Read the model definition and answer for the solid it produces. Units are mm, in the model's axes. A direction names the side the tool comes from. Give positions to 0.01 mm unless a question says otherwise; leave off trailing zeros. Write each loop counter-clockwise with the first axis right and the second up, starting at its lowest first coordinate (ties: lowest second). Pieces come first, ordered by that corner, then holes. Notation, with made-up numbers: (35, 9) - (65, 9) arc R13 ccw to (65, 16) - close; hole circle Ø3 at (-34, 65.5). An arc over 180 degrees is marked (long way). Answer as CSV lines item,"result".
```python
from build123d import *

# Parameters (mm, degrees)
CROQUIS1_W              = 25.4
CROQUIS1_H              = 11.3
SALIENTE_EXTRUIR1_DEPTH = 11.7
CROQUIS2_W              = 5.25
CROQUIS2_H              = 11.7
CORTAR_EXTRUIR1_DEPTH   = 8.3
CROQUIS3_W              = 11.9
CROQUIS3_H              = 9.8
CORTAR_EXTRUIR2_DEPTH   = 31.161896492
CROQUIS4_R              = 1
CORTAR_EXTRUIR3_DEPTH   = 30.170875887


with BuildPart() as part:
    # Croquis1 → Saliente-Extruir1 (new body)
    with BuildSketch(Plane.XY):
        with Locations((12.7, 5.65)):
            Rectangle(CROQUIS1_W, CROQUIS1_H)
    extrude(amount=SALIENTE_EXTRUIR1_DEPTH)

    # Croquis2 → Cortar-Extruir1 (cut)
    with BuildSketch(Plane(origin=(0, 11.3, 0), x_dir=(1, 0, 0), z_dir=(0, 1, 0))):
        with Locations((2.625, -5.85)):
            Rectangle(CROQUIS2_W, CROQUIS2_H)
        with Locations((22.775, -5.85)):
            Rectangle(CROQUIS2_W, CROQUIS2_H)
    extrude(amount=-CORTAR_EXTRUIR1_DEPTH, mode=Mode.SUBTRACT)

    # Croquis3 → Cortar-Extruir2 (cut, through all)
    with BuildSketch(Plane.XY.offset(11.7)):
        with Locations((12.7, 4.9)):
            Rectangle(CROQUIS3_W, CROQUIS3_H)
    extrude(amount=-CORTAR_EXTRUIR2_DEPTH, mode=Mode.SUBTRACT)

    # Croquis4 → Cortar-Extruir3 (cut, through all)
    with BuildSketch(Plane(origin=(0, 3, 0), x_dir=(1, 0, 0), z_dir=(0, 1, 0))):
        with Locations(Location((21.2, -4.7, 0), (0, 0, 270))):
            Circle(CROQUIS4_R)
        with Locations(Location((4.2, -4.7, 0), (0, 0, 270))):
            Circle(CROQUIS4_R)
    extrude(amount=-CORTAR_EXTRUIR3_DEPTH, mode=Mode.SUBTRACT)


solid = part.part
```
(1) A cutting plane is placed at D-D (z = 1.75). Write down the section's boundary in (x, y).
Worked out:
outline,"(0, 0) - (6.75, 0) - (6.75, 9.8) - (18.65, 9.8) - (18.65, 0) - (25.4, 0) - (25.4, 3) - (20.15, 3) - (20.15, 11.3) - (5.25, 11.3) - (5.25, 3) - (0, 3) - close"
(2) A cutting plane is placed at C-C (y = 7.5). Write down the section's boundary in (x, z), and give its area (3 significant figures).
Worked out:
outline,"(5.25, 0) - (6.75, 0) - (6.75, 11.7) - (5.25, 11.7) - close; (18.65, 0) - (20.15, 0) - (20.15, 11.7) - (18.65, 11.7) - close"
area,"35.1 mm^2"
(3) Each of these flat-tipped pins is pushed along its axis until it touches: P1, Ø2, axis at x = 17, y = 1.5, coming from the -Z side; P2, Ø1.5, axis at y = 5.5, z = 8, coming from the -X side; P3, Ø4, axis at x = 23, z = 7, coming from the +Y side; P4, Ø6, axis at x = 15, z = 5, coming from the -Y side. Where does it stop, or does it pass through?
Worked out:
P1,"passes through"
P2,"stops at x = 5.25"
P3,"stops at y = 3"
P4,"stops at y = 9.8"
(4) For faces 1 (the flat face through (13, 11.3, 6)), 2 (the flat face through (3, 3, 6)), 3 (the flat face through (23, 3, 6)), 4 (the flat face through (13, 9.8, 6)), determine the directions among +Z, -Z, +X, -X, +Y, -Y from which every point of the face is accessible in a straight line to the end or side of a thin tool.
Worked out:
face 1,"+Z, -Z, +X, -X, +Y"
face 2,"+Z, -Z, -X, +Y"
face 3,"+Z, -Z, +X, +Y"
face 4,"+Z, -Z, -Y"
(5) Find the intervals of material crossed by L1, parallel to X at y = 1, z = 4.7; L2, parallel to X at y = 6, z = 1.5; L3, parallel to X at y = 2, z = 5.75, in increasing order.
Worked out:
L1,"x = 0 to 3.2, 5.2 to 6.75, 18.65 to 20.2, 22.2 to 25.4"
L2,"x = 5.25 to 6.75, 18.65 to 20.15"
L3,"x = 0 to 6.75, 18.65 to 25.4"
(6) A cutting plane is placed at A-A (x = 21.2). Write down the section's boundary in (y, z).
Worked out:
outline,"(0, 0) - (3, 0) - (3, 3.7) - (0, 3.7) - close; (0, 5.7) - (3, 5.7) - (3, 11.7) - (0, 11.7) - close"
(7) A cutting plane is placed at B-B (z = 4.7). Write down the section's boundary in (x, y).
Worked out:
outline,"(0, 0) - (3.2, 0) - (3.2, 3) - (0, 3) - close; (5.2, 0) - (6.75, 0) - (6.75, 9.8) - (18.65, 9.8) - (18.65, 0) - (20.2, 0) - (20.2, 3) - (20.15, 3) - (20.15, 11.3) - (5.25, 11.3) - (5.25, 3) - (5.2, 3) - close; (22.2, 0) - (25.4, 0) - (25.4, 3) - (22.2, 3) - close"
(8) The mould has two halves that part along X. Classify faces 5 (the flat face through (3, 0, 6)), 6 (the cylindrical face through (3.224, 1.521, 4.483)), 7 (the flat face through (20.15, 7, 6)): +X half, -X half, draft (parallel to the pull), parting line (faces both ways), or undercut.
Worked out:
face 5,"draft"
face 6,"undercut"
face 7,"+X half"
